Autodesk Inventor part; units mm, degrees
ref_plane "YZ Plane" through (0, 0, 0) normal (1, 0, 0) x (0, 1, 0)
ref_plane "XZ Plane" through (0, 0, 0) normal (0, 1, 0) x (-1, 0, 0)
ref_plane "XY Plane" through (0, 0, 0) normal (0, 0, 1) x (1, 0, 0)
sketch "Sketch1" plane through (0, 0, 0) normal (1, 0, 0) x (0, 1, 0)
  line L0 (0, 0) -> (29.1856, 16.8503)
  line L1 (29.1856, 16.8503) -> (49.5056, -18.345)
  line L2 (0, -73.2789) -> (0, 37.3579)
  line L3 (49.5056, -18.345) -> (0, -46.927)
  line L4 (0, 0) -> (0, -46.927)
  line L5 (32.9956, 10.2512) -> (0, -8.7988) construction
  dimension "d0" = 40.64
  dimension "d1" = 60
  dimension "d5" = 7.62
  dimension "d6" = 38.1
extrude "Extrusion1" add sketch "Sketch1" along normal mid plane 40.64
sketch "Sketch2" plane through (-20.32, 29.1856, 16.8503) normal (0, 0.866, 0.5) x (1, 0, 0)
  line L0 (0, 0) -> (40.64, 0) construction
  line L1 (40.64, 0) -> (40.64, 40.64) construction
  line L2 (0, 0) -> (40.64, 40.64) construction
  line L3 (40.64, 40.64) -> (0, 40.64) construction
  line L4 (0, 40.64) -> (40.64, 0) construction
  line L5 (7.62, 7.62) -> (33.02, 7.62)
  line L6 (33.02, 7.62) -> (33.02, 33.02)
  line L7 (33.02, 33.02) -> (7.62, 33.02)
  line L8 (7.62, 33.02) -> (7.62, 7.62)
  line L9 (7.62, 7.62) -> (33.02, 33.02) construction
  line L10 (33.02, 7.62) -> (7.62, 33.02) construction
  point P0 (20.32, 0)
  point P1 (20.32, 20.32)
  dimension "d7" = 25.4
extrude "Extrusion2" cut sketch "Sketch2" against normal blind 38.1
sketch "Sketch3" plane through (0, 0, 0) normal (1, 0, 0) x (0, 1, 0)
  line L0 (29.1856, 16.8503) -> (0, 0)
  line L1 (0, 0) -> (0, -46.927)
  line L2 (0, -46.927) -> (49.5056, -18.345)
  line L3 (12.7, -30.7959) -> (0, -8.7988)
  line L4 (32.9956, 10.2512) -> (0, -8.7988)
  line L5 (0, 0) -> (0, -46.927)
  line L6 (29.1856, 16.8503) -> (15.6348, 16.8503) construction
  line L7 (0, 0) -> (29.1856, 16.8503)
  line L8 (0, 0) -> (0, 42.2503)
  line L9 (49.5056, -18.345) -> (0, -46.927)
  line L10 (0, -46.927) -> (0, -72.327)
  line L11 (0, -108.8389) -> (0, 72.9179)
  line L12 (0, 42.2503) -> (-12.7, 42.2503)
  line L13 (-12.7, 42.2503) -> (-12.7, -72.327)
  line L14 (-12.7, -72.327) -> (0, -72.327)
  point P0 (1.0999, -13.335)
  point P1 (0, -8.7988)
  dimension "d10" = 25.4
  dimension "d11" = 25.4
  dimension "d12" = 12.7
extrude "Extrusion3" add sketch "Sketch3" along normal mid plane 22.86
equation "\"d0\" = widthToSupportExtrusion"
equation "\"d1\" = attachementAngle"
equation "\"d6\" = insertDepth"
equation "\"d2\" = widthToSupportExtrusion"
equation "\"d7\" = extrusionSize"
equation "\"d8\" = insertDepth"
equation "\"d12\" = supportBaseDepth"
equation "\"d13\" = supportBaseWidth"
equation "\"attachementAngle\" = 60deg"
equation "\"extrusionSize\" = 25.4"
equation "\"wallThickness\" = 6.35"
equation "\"slipClearance\" = 1.27"
equation "\"insertForExtrusion\" = extrusionSize + 2 * slipClearance"
equation "\"widthToSupportExtrusion\" = insertForExtrusion + 2 * wallThickness"
equation "\"insertDepth\" = 38.1"
equation "\"supportBaseWidth\" = 22.86"
equation "\"supportBaseDepth\" = 12.7"
properties part number "60DegreeAttachementV02"
Build history of the part. All positions in model axes, mm. A direction names the side the tool comes from. Give positions to 0.01 mm unless a question says otherwise; leave off trailing zeros. Loops run counter-clockwise (first coordinate to the right, second up) from the corner with the lowest first, then second, coordinate; pieces in that order, holes last. Notation, with made-up numbers: (10.5, 45.5) -> (36.5, 45.5) arc R24 cw to (36.5, 71.5) -> close; hole circle Ø10 at (81, 15). An arc over 180 degrees is marked (long way). Answer in a Markdown table with one row per item.
Item 1: Flat gauge pins, fed straight in: P1, Ø7, axis at x = -1.5, z = 23, coming from the +Y side; P2, Ø6.5, axis at y = -8.5, z = -22, coming from the +X side; P3, Ø18.5, axis at x = -2.5, z = -55, coming from the +Y side; P4, Ø10, axis at x = -14.5, z = -28, coming from the -Y side. Where does each tip first touch, or does it go through?
Findings below:
| item | result |
|---|---|
| P1 | stops at y = 0 |
| P2 | stops at x = 11.43 |
| P3 | stops at y = 2.04 |
| P4 | stops at y = -12.7 |
Item 2: Probe line 1 along X through (y, z) = (-4.5, -54); line 2 along Z through (x, y) = (-9, 1); line 3 along Y through (x, z) = (5, -56). List the from-to ranges inside material, lowest first. Write a range as [from, to].
Findings below:
| item | result |
|---|---|
| line 1 | x = [-11.43, 11.43] |
| line 2 | z = [-46.35, -10.53], [-8.22, 0.58] |
| line 3 | y = [-12.7, 0] |
Item 3: Tool access for faces 1 (the flat face through (11.43, -6, -14)), 2 (the flat face through (-0.178, 6.438, -19.954)), 3 (the flat face through (-0.18, 16.73, 0.86)), 4 (the flat face through (0, 0, -59)): list every direction of +Z, -Z, +X, -X, +Y, -Y with a clear straight run to the whole face (end or side of a thin tool).
Findings below:
| item | result |
|---|---|
| face 1 | +Z, -Z, +X, -Y |
| face 2 | none |
| face 3 | +Y |
| face 4 | -Z, +X, -X, +Y |
Item 4: Slice it at A-A on y = 18. Write the cut outline in (x, z).
Findings below:
| item | result |
|---|---|
| outline | (-20.32, -36.53) -> (20.32, -36.53) -> (20.32, 10.39) -> (-20.32, 10.39) -> close; hole (-12.7, -27.74) -> (12.7, -27.74) -> (12.7, 1.59) -> (-12.7, 1.59) -> close |
Item 5: Mould opens along X. For faces 5 (the flat face through (0.178, 29.428, -21.138)), 6 (the flat face through (0, 0, 21)), 7 (the flat face through (20.32, 19, -15)) say: pulls with the +X half, pulls with the -X half, needs draft (parallel to the pull), parting line crosses it, or undercut.
Findings below:
| item | result |
|---|---|
| face 5 | undercut |
| face 6 | needs draft |
| face 7 | pulls with the +X half |
Item 6: Slice it at D-D on y = 37.5. Write the cut outline in (x, z).
Findings below:
| item | result |
|---|---|
| outline | (-20.32, -25.28) -> (20.32, -25.28) -> (20.32, 2.45) -> (12.7, 2.45) -> (12.7, -16.48) -> (-12.7, -16.48) -> (-12.7, 2.45) -> (-20.32, 2.45) -> close |
Item 7: Slice it at B-B on z = -16.5. Write the cut outline in (x, y), plus the area to 3 significant figures.
Findings below:
| item | result |
|---|---|
| outline | (-20.32, 0) -> (-11.43, 0) -> (-11.43, -12.7) -> (11.43, -12.7) -> (11.43, 0) -> (20.32, 0) -> (20.32, 48.44) -> (-20.32, 48.44) -> close; hole (-12.7, 4.44) -> (12.7, 4.44) -> (12.7, 37.46) -> (-12.7, 37.46) -> close |
| area | 1,420 mm² |
